Could you check a few things on this model? Use its own coordinates, in mm. Give positions to 0.01 mm unless a question says otherwise; leave off trailing zeros. Order: outer loops, then holes, each group sorted by start corner. A loop starts at its lowest first (then second) coordinate and runs counter-clockwise, first axis right, second up. Notation, with made-up numbers: M 18,18 L 73,18 A27 ccw 73,53 Z; hole C 61,38 d6. An arc over 180 degrees is marked long. Return JSON: item names as keys, results as strings. Group by question number.
```python
from build123d import *

# Parameters (mm, degrees)
F0_R     = 80
F1_DEPTH = 2
F2_R     = 25
F3_DEPTH = 25.4
F4_R     = 2
F5_DEPTH = 25.4
F7_DEPTH = 25.4


with BuildPart() as f1:
    # F0 (on Top) → F1 (new body)
    with BuildSketch(Plane.XY):
        Circle(F0_R)
    extrude(amount=F1_DEPTH)

    # F2 (on face) → F3 (cut)
    with BuildSketch(Plane.XY.offset(2)):
        with Locations((42.711879087, -67.6438865298)):
            Circle(F2_R)
    extrude(amount=-F3_DEPTH, mode=Mode.SUBTRACT)

    # F4 (on face) → F5 (cut)
    with BuildSketch(Plane.XY.offset(2)):
        Circle(F4_R)
    extrude(amount=-F5_DEPTH, mode=Mode.SUBTRACT)

    # F6 (on face) → F7 (cut)
    with BuildSketch(Plane.XY.offset(2)):
        with BuildLine():
            ThreePointArc((-43.8903481832, 66.8852549996), (-15.8440218297, 52.7258990739), (3.8976538135, 77.166644254))
            ThreePointArc((3.8976538135, 77.166644254), (3.8598196829, 78.5415170144), (3.7464318049, 79.9122284055))
            ThreePointArc((3.7464318049, 79.9122284055), (-21.1023461865, 77.166644254), (-43.8903481832, 66.8852549996))
        make_face()
        with BuildLine():
            ThreePointArc((-43.8903481832, 66.8852549996), (-21.1023461865, 77.166644254), (3.7464318049, 79.9122284055))
            ThreePointArc((3.7464318049, 79.9122284055), (-27.6968293698, 101.2812205834), (-43.8903481832, 66.8852549996))
        make_face()
    extrude(amount=-F7_DEPTH, mode=Mode.SUBTRACT)


solid = f1.part
```
1. If we mould it in two halves opening along Y, with no side actions, what happens to faces 1 (the cylindrical face through (0, -2, 1)), 2 (the cylindrical face through (-73.83, -30.81, 0.99)), 3 (the flat face through (-1, -17, 0))? For each: pulls with the +Y half, pulls with the -Y half, needs draft (parallel to the pull), parting line crosses it, or undercut.
2. I need wall thicknesses on L1, parallel to Y at x = 0, z = 1.3; L2, parallel to X at y = -45.5, z = 0.95; L3, parallel to X at y = 61, z = 1.5. Which ranges of each line are inside material? Lowest first, please. Write a range as from..to.
3. For pin 1 (1 mm diameter, centred on x = -27.5, z = 1, fed in from -Y); pin 2 (3 mm diameter, centred on x = 0, y = 0, fed in from -Z), each with a flat end and sliding along its axis, tell me the tip position at first contact or that it passes through.
4. Imagine slicing it at A-A, the plane y = 0. Please give me the cut outline in (x, z).
5. Imagine slicing it at C-C, the plane z = 0.95. Please give me the cut outline in (x, y), plus the area to 3 significant figures.
6. Imagine slicing it at D-D, the plane x = -48.5. Please give me the cut outline in (y, z), plus the area to 3 significant figures.
7. Imagine slicing it at B-B, the plane x = 0. Please give me the cut outline in (y, z).
Values:
{
 "1": {"face 1": "undercut", "face 2": "parting line crosses it", "face 3": "needs draft"},
 "2": {"L1": "y = -80..-2, 2..63.76", "L2": "x = -65.8..31.11, 54.32..65.8", "L3": "x = -51.76..-40.17, -2.03..51.76"},
 "3": {"pin 1": "stops at y = -75.31", "pin 2": "passes through"},
 "4": {"outline": "M -80,0 L -2,0 L -2,2 L -80,2 Z; M 2,0 L 80,0 L 80,2 L 2,2 Z"},
 "5": {"outline": "M -43.89,66.89 A80 ccw 19.75,-77.52 A25 cw 61.51,-51.16 A80 ccw 3.75,79.91 A25 cw Z; hole C 0,0 d4", "area": "18,300 mm²"},
 "6": {"outline": "M -63.62,0 L 63.62,0 L 63.62,2 L -63.62,2 Z", "area": "254 mm²"},
 "7": {"outline": "M -80,0 L -2,0 L -2,2 L -80,2 Z; M 2,0 L 63.76,0 L 63.76,2 L 2,2 Z"}
}
